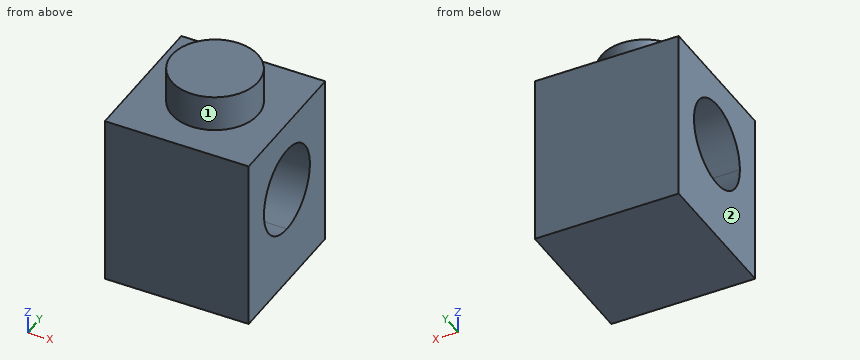
from build123d import *

# Parameters (mm, degrees)
F0_W     = 8
F0_H     = 8
F1_DEPTH = 9.6
F3_DEPTH = 25
F4_R     = 2.4
F5_DEPTH = 2


with BuildPart() as f1:
    # F0 (on Top) → F1 (new body)
    with BuildSketch(Plane.XY):
        with Locations((-0.409037, 0.409032)):
            Rectangle(F0_W, F0_H)
    extrude(amount=F1_DEPTH)

    # F2 (on face) → F3 (cut)
    with BuildSketch(Plane(origin=(-4.409037, 0, 0), x_dir=(0, -1, 0), z_dir=(-1, 0, 0))):
        with BuildLine():
            ThreePointArc((1.990968, 5.6), (-2.106088, 7.297056), (-0.409032, 3.2))
            ThreePointArc((-0.409032, 3.2), (1.288024, 3.902944), (1.990968, 5.6))
        make_face()
    extrude(amount=-F3_DEPTH, mode=Mode.SUBTRACT)

    # F4 (on face) → F5 (join)
    with BuildSketch(Plane.XY.offset(9.6)):
        with Locations((-0.409037, 0.409032)):
            Circle(F4_R)
    extrude(amount=F5_DEPTH)


solid = f1.part
Geometry check sheet. Reference: the model listing, model coordinates, mm. Face numbers are marked on the shaded views. A direction names the side the tool comes from. Give positions to 0.01 mm unless a question says otherwise; leave off trailing zeros. Order: outer loops, then holes, each group sorted by start corner. A loop starts at its lowest first (then second) coordinate and runs counter-clockwise, first axis right, second up.
1. Sectioned sample at C-C (x = 0.5). Record the boundary of the cut face in (y, z), then the cut area to 3 significant figures.
Completed:
outline: (-3.59, 0) - (4.41, 0) - (4.41, 9.6) - (2.63, 9.6) - (2.63, 11.6) - (-1.81, 11.6) - (-1.81, 9.6) - (-3.59, 9.6) - close; hole (-1.99, 5.6) arc R2.4 ccw to (0.41, 3.2) arc R2.4 ccw (long way) to start
area: 67.6 mm2
2. Sectioned sample at D-D (z = 6.25). Record the boundary of the cut face in (x, y).
Completed:
outline: (-4.41, -3.59) - (3.59, -3.59) - (3.59, -1.9) - (-4.41, -1.9) - close; (-4.41, 2.72) - (3.59, 2.72) - (3.59, 4.41) - (-4.41, 4.41) - close
3. Sectioned sample at A-A (z = 4.5). Record the boundary of the cut face in (x, y).
Completed:
outline: (-4.41, -3.59) - (3.59, -3.59) - (3.59, -1.72) - (-4.41, -1.72) - close; (-4.41, 2.54) - (3.59, 2.54) - (3.59, 4.41) - (-4.41, 4.41) - close
4. Scan lines: line 1 (Y direction, x = -1, z = 5.6); line 2 (Z direction, x = -0.5, y = -2.5); line 3 (Y direction, x = 1, z = 5). Record each from-to range of solid material in increasing order.
Completed:
line 1: y = -3.59 to -1.99, 2.81 to 4.41
line 2: z = 0 to 9.6
line 3: y = -3.59 to -1.91, 2.73 to 4.41
5. Sectioned sample at B-B (y = -0.75). Record the boundary of the cut face in (x, z), then the cut area to 3 significant figures.
Completed:
outline: (-4.41, 0) - (3.59, 0) - (3.59, 3.5) - (-4.41, 3.5) - close; (-4.41, 7.7) - (3.59, 7.7) - (3.59, 9.6) - (1.69, 9.6) - (1.69, 11.6) - (-2.51, 11.6) - (-2.51, 9.6) - (-4.41, 9.6) - close
area: 51.6 mm2
6. Access from +Z, -Z, +X, -X, +Y, -Y to the whole of each face (thin tool, end or side, straight path). Record for the marked faces 1 and 2.
Completed:
face 1: +Z
face 2: +Z, -Z, -X, +Y, -Y
